```python
from build123d import *

# Parameters (mm, degrees)
SKETCH_1_W          = 30
SKETCH_1_H          = 20
EXTRUDE_1_DEPTH     = 4.2
SKETCH_2_R          = 3.05
CUT_EXTRUDE_1_DEPTH = 19.510537539
SKETCH_3_W          = 8
SKETCH_3_H          = 8.5
CUT_EXTRUDE_2_DEPTH = 19.510537539
EXTRUDE_2_DEPTH     = 2
SKETCH_5_R          = 1.75
CUT_EXTRUDE_3_DEPTH = 19.510537539
SKETCH_6_W          = 8
SKETCH_6_H          = 2
CUT_EXTRUDE_4_DEPTH = 20.064102392
SKETCH_7_R          = 1.1
CUT_EXTRUDE_5_DEPTH = 20.064102392
SKETCH_8_W          = 2.8
SKETCH_8_H          = 2.8
EXTRUDE_3_DEPTH     = 3
SKETCH_9_R          = 3.05
SKETCH_9_R_2        = 1.75
EXTRUDE_4_DEPTH     = 3.8


with BuildPart() as part:
    # 草图1 → 凸台-拉伸1 (new body)
    with BuildSketch(Plane(origin=(0, 0, 0), x_dir=(1, 0, 0), z_dir=(0, 1, 0))):
        Rectangle(SKETCH_1_W, SKETCH_1_H)
    extrude(amount=EXTRUDE_1_DEPTH)

    # 草图2 → 切除-拉伸1 (cut, through all)
    with BuildSketch(Plane(origin=(0, 4.2, 0), x_dir=(1, 0, 0), z_dir=(0, 1, 0))):
        with Locations(Location((-7.5, 3, 0), (0, 0, 270))):
            Circle(SKETCH_2_R)
        with Locations(Location((7.5, 3, 0), (0, 0, 270))):
            Circle(SKETCH_2_R)
    extrude(amount=-CUT_EXTRUDE_1_DEPTH, mode=Mode.SUBTRACT)

    # 草图3 → 切除-拉伸2 (cut, through all)
    with BuildSketch(Plane(origin=(0, 4.2, 0), x_dir=(1, 0, 0), z_dir=(0, 1, 0))):
        with Locations((0, -5.75)):
            Rectangle(SKETCH_3_W, SKETCH_3_H)
    extrude(amount=-CUT_EXTRUDE_2_DEPTH, mode=Mode.SUBTRACT)

    # 草图4 → 凸台-拉伸2 (add)
    with BuildSketch(Plane(origin=(0, 4.2, 0), x_dir=(1, 0, 0), z_dir=(0, 1, 0))):
        Polygon((-4, -1.5), (4, -1.5), (4, -10), (15, -10), (15, 10), (-15, 10), (-15, -10), (-4, -10), align=None)
    extrude(amount=EXTRUDE_2_DEPTH)

    # 草图5 → 切除-拉伸3 (cut, through all)
    with BuildSketch(Plane.XZ.offset(-4.2)):
        with Locations(Location((-7.5, -3, 0), (0, 0, 270))):
            Circle(SKETCH_5_R)
        with Locations(Location((7.5, -3, 0), (0, 0, 270))):
            Circle(SKETCH_5_R)
    extrude(amount=-CUT_EXTRUDE_3_DEPTH, mode=Mode.SUBTRACT)

    # 草图6 → 切除-拉伸4 (cut, through all)
    with BuildSketch(Plane(origin=(0, 6.2, 0), x_dir=(1, 0, 0), z_dir=(0, 1, 0))):
        with Locations((0, 9)):
            Rectangle(SKETCH_6_W, SKETCH_6_H)
    extrude(amount=-CUT_EXTRUDE_4_DEPTH, mode=Mode.SUBTRACT)

    # 草图7 → 切除-拉伸5 (cut, through all)
    with BuildSketch(Plane(origin=(0, 6.2, 0), x_dir=(1, 0, 0), z_dir=(0, 1, 0))):
        with Locations(Location((-7, -6, 0), (0, 0, 270))):
            Circle(SKETCH_7_R)
        with Locations(Location((7, -6, 0), (0, 0, 90))):
            Circle(SKETCH_7_R)
    extrude(amount=-CUT_EXTRUDE_5_DEPTH, mode=Mode.SUBTRACT)

    # 草图8 → 凸台-拉伸3 (add)
    with BuildSketch(Plane.XZ):
        with Locations((0, -5)):
            Rectangle(SKETCH_8_W, SKETCH_8_H)
    extrude(amount=EXTRUDE_3_DEPTH)

    # 草图9 → 凸台-拉伸4 (add)
    # profile 1 of 2: a face of its own
    with BuildSketch(Plane.XZ.offset(-4.2)):
        with Locations(Location((7.5, -3, 0), (0, 0, 90))):
            Circle(SKETCH_9_R)
        with Locations(Location((7.5, -3, 0), (0, 0, 270))):
            Circle(SKETCH_9_R_2, mode=Mode.SUBTRACT)
    # profile 2 of 2: a face of its own
    with BuildSketch(Plane.XZ.offset(-4.2)):
        with Locations(Location((-7.5, -3, 0), (0, 0, 90))):
            Circle(SKETCH_9_R)
        with Locations(Location((-7.5, -3, 0), (0, 0, 270))):
            Circle(SKETCH_9_R_2, mode=Mode.SUBTRACT)
    extrude(amount=EXTRUDE_4_DEPTH)


solid = part.part
```
Source: CAD feature listing. Evaluate the final solid. Frame: model axes, mm. A direction names the side the tool comes from. Give positions to 0.01 mm unless a question says otherwise; leave off trailing zeros. Loops run counter-clockwise (first coordinate to the right, second up) from the corner with the lowest first, then second, coordinate; pieces in that order, holes last. Notation, with made-up numbers: (12, 31) - (37, 31) arc R28 ccw to (37, 52) - close; hole circle Ø2 at (72.5, -17.75). An arc over 180 degrees is marked (long way). Use CSV: the item, a comma, the result in double quotes.
1) Pin query (flat end, axial travel): P1, Ø8, axis at x = -6, z = 4.5, coming from the -Y side; P2, Ø4, axis at x = 7.5, z = -3, coming from the -Y side; P3, Ø1.8, axis at x = 7, z = 6, coming from the -Y side; P4, Ø1.4, axis at x = 0.5, y = -1.5, coming from the +Z side. Return the tip coordinate at first contact, or that it passes through.
Worked out:
P1,"stops at y = 0"
P2,"stops at y = 0.4"
P3,"passes through"
P4,"stops at z = -3.6"
2) Line query: line 1 (X direction, y = 1.3, z = -3); line 2 (X direction, y = 1.5, z = 6); line 3 (X direction, y = 0.75, z = 8.5). Output: solid intervals per line, ascending.
Worked out:
line 1,"x = -15 to -9.25, -5.75 to 5.75, 9.25 to 15"
line 2,"x = -15 to -8.1, -5.9 to -4, 4 to 5.9, 8.1 to 15"
line 3,"x = -15 to -4, 4 to 15"
3) Cut plane C-C (y = 3.5). Output: boundary loops of the cut face in (x, z), and give its area (3 significant figures).
Worked out:
outline,"(-15, -10) - (-4, -10) - (-4, -8) - (4, -8) - (4, -10) - (15, -10) - (15, 10) - (4, 10) - (4, 1.5) - (-4, 1.5) - (-4, 10) - (-15, 10) - close; hole circle Ø3.5 at (-7.5, -3); hole circle Ø2.2 at (-7, 6); hole circle Ø3.5 at (7.5, -3); hole circle Ø2.2 at (7, 6)"
area,"489 mm^2"
4) Mould query, pull axis X, two halves, no side actions, for faces 1 (the flat face through (-1.4, -1, -5)), 2 (the cylindrical face through (7.421, 3.143, 4.984)), 3 (the flat face through (0, -3, -5)), 4 (the flat face through (1.4, -1, -5)). Classes: +X half, -X half, draft (parallel to the pull), parting line (faces both ways), or undercut.
Worked out:
face 1,"-X half"
face 2,"undercut"
face 3,"draft"
face 4,"+X half"
5) Cut plane D-D (x = -1). Output: boundary loops of the cut face in (y, z), and give its area (3 significant figures).
Worked out:
outline,"(-3, -6.4) - (0, -6.4) - (0, -8) - (6.2, -8) - (6.2, 1.5) - (0, 1.5) - (0, -3.6) - (-3, -3.6) - close"
area,"67.3 mm^2"
6) Set-up query: faces 5 (the flat face through (-4, 3, 6)), 6 (the cylindrical face through (7.634, 0.203, -6.047)), 7 (the flat face through (-4, 3, -9)), 8 (the flat face through (0, 6.2, 0)). Return all of +Z, -Z, +X, -X, +Y, -Y with unobstructed straight access to the full face (end or side cutting, diameter ignored); none if empty.
Worked out:
face 5,"+Z, +Y, -Y"
face 6,"-Y"
face 7,"-Z, +Y, -Y"
face 8,"+Z, -Z, +X, -X, +Y"
7) Cut plane B-B (z = -3). Output: boundary loops of the cut face in (x, y), and give its area (3 significant figures).
Worked out:
outline,"(-15, 0) - (-10.55, 0) - (-10.55, 0.4) - (-9.25, 0.4) - (-9.25, 6.2) - (-15, 6.2) - close; (-5.75, 0.4) - (-4.45, 0.4) - (-4.45, 0) - (4.45, 0) - (4.45, 0.4) - (5.75, 0.4) - (5.75, 6.2) - (-5.75, 6.2) - close; (9.25, 0.4) - (10.55, 0.4) - (10.55, 0) - (15, 0) - (15, 6.2) - (9.25, 6.2) - close"
area,"141 mm^2"
8) Cut plane A-A (z = 4.5). Output: boundary loops of the cut face in (x, y), and give its area (3 significant figures).
Worked out:
outline,"(-15, 0) - (-4, 0) - (-4, 6.2) - (-15, 6.2) - close; (4, 0) - (15, 0) - (15, 6.2) - (4, 6.2) - close"
area,"136 mm^2"
